Autodesk Inventor part; units mm, degrees
ref_plane "YZ Plane" through (0, 0, 0) normal (1, 0, 0) x (0, 1, 0)
ref_plane "XZ Plane" through (0, 0, 0) normal (0, 1, 0) x (-1, 0, 0)
ref_plane "XY Plane" through (0, 0, 0) normal (0, 0, 1) x (1, 0, 0)
sketch "Sketch3" plane through (0, 0, 0) normal (0, 0, 1) x (1, 0, 0)
  line L0 (0, 0) -> (-55.38, 0)
  line L1 (-55.38, 0) -> (-55.38, 47.03)
  line L2 (-55.38, 47.03) -> (0, 47.03)
  line L3 (0, 47.03) -> (0, 0)
  line L4 (5, -5) -> (5, 52.03)
  line L5 (5, 52.03) -> (-60.38, 52.03)
  line L6 (5, -5) -> (-60.38, -5)
  line L7 (-60.38, -5) -> (-60.38, 52.03)
  dimension "d26" = 47.03
  dimension "d27" = 55.38
extrude "Extrusion10" add sketch "Sketch3" along normal blind 10
sketch "Sketch10" plane through (0, 0, 10) normal (0, 0, 1) x (1, 0, 0)
  line L0 (-60.38, 52.03) -> (5, 52.03)
  line L1 (5, 52.03) -> (5, -5)
  line L2 (5, -5) -> (-60.38, -5)
  line L3 (-60.38, -5) -> (-60.38, 52.03)
  point P0 (0, 0)
extrude "Extrusion11" add sketch "Sketch10" along normal blind 5
sketch "Sketch11" plane through (0, 0, 15) normal (0, 0, 1) x (1, 0, 0)
  line L0 (5, -5) -> (-0.19, -5)
  line L1 (-0.19, -5) -> (-0.19, -3.985)
  line L2 (-0.19, -5) -> (0.825, -5) construction
  line L3 (-0.19, -3.985) -> (-55.19, -3.985)
  line L4 (-55.19, -3.985) -> (-55.19, 51.015)
  line L5 (-55.19, 51.015) -> (-0.19, 51.015)
  line L6 (-0.19, 51.015) -> (-0.19, -3.985)
  point P0 (0, 0)
  point P1 (-60.38, -5)
  point P2 (-60.38, 52.03)
  dimension "d73" = 65.38
  dimension "d76" = 5.19
  dimension "d78" = 1.015
  dimension "d79" = 90
  dimension "d80" = 55
  dimension "d81" = 55
extrude "Extrusion12" cut sketch "Sketch11" against normal blind 2
properties part number "End-Effector"
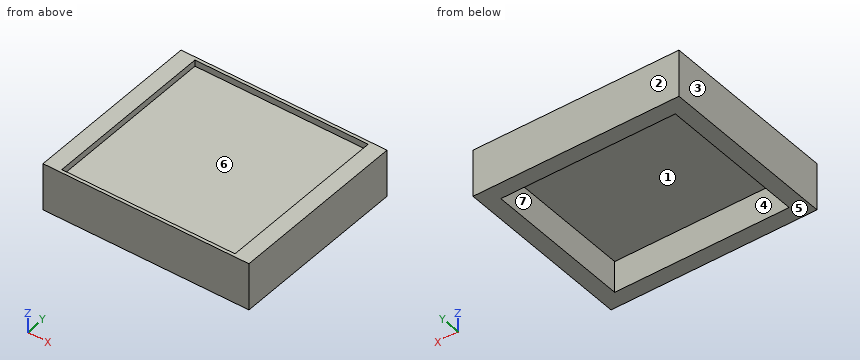
Work out the finished part from the listing and answer in its coordinate system (mm). Face numbers are marked on the shaded views. A direction names the side the tool comes from. Round coordinates to 2 decimals unless told otherwise and drop trailing zeros. Write each loop counter-clockwise with the first axis right and the second up, starting at its lowest first coordinate (ties: lowest second). Pieces come first, ordered by that corner, then holes.
1) A tool of negligible diameter and unlimited length cuts with its end or side. For the marked faces 5, 6 and 7, from which of +Z, -Z, +X, -X, +Y, -Y can it reach the whole face along a straight path? Write none if from no direction.
2) A cutting plane is placed at B-B (y = 28). Give the vertices of the cut face in (x, z), plus the area to 3 significant figures.
3) Given pin 1 Ø8 at (x, y) = (-6.5, 29.5) entering from -Z, flat-ended and moving along its own axis, determine where the tip first touches the part or whether it passes through.
4) Straight lines are drawn through the part: line 1 (Y direction, x = -46, z = 6); line 2 (X direction, y = 21, z = 3.5); line 3 (Z direction, x = -38, y = 4). For each, find the intervals that lie inside material, in ascending order.
5) A cutting plane is placed at A-A (z = 5.25). Give the vertices of the cut face in (x, y).
6) A cutting plane is placed at C-C (x = -54). Give the vertices of the cut face in (y, z) (3 decimals).
7) The mould has two halves that part along X. Classify the marked faces 1, 2, 3 and 4: pulls with the +X half, pulls with the -X half, needs draft (parallel to the pull), parting line crosses it, or undercut.
Completed:
1. face 5: -Z, +X, -X, +Y, -Y
1. face 6: +Z
1. face 7: -Z
2. outline: (-60.38, 0) - (-55.38, 0) - (-55.38, 10) - (0, 10) - (0, 0) - (5, 0) - (5, 15) - (-0.19, 15) - (-0.19, 13) - (-55.19, 13) - (-55.19, 15) - (-60.38, 15) - close
2. area: 317 mm2
3. pin 1: stops at z = 10
4. line 1: y = -5 to 0, 47.03 to 52.03
4. line 2: x = -60.38 to -55.38, 0 to 5
4. line 3: z = 10 to 13
5. outline: (-60.38, -5) - (5, -5) - (5, 52.03) - (-60.38, 52.03) - close; hole (-55.38, 0) - (0, 0) - (0, 47.03) - (-55.38, 47.03) - close
6. outline: (-5, 0) - (0, 0) - (0, 10) - (47.03, 10) - (47.03, 0) - (52.03, 0) - (52.03, 15) - (51.015, 15) - (51.015, 13) - (-3.985, 13) - (-3.985, 15) - (-5, 15) - close
7. face 1: undercut
7. face 2: needs draft
7. face 3: pulls with the -X half
7. face 4: undercut
